from build123d import *

# Parameters (mm, degrees)
EXTRUDE_1_DEPTH     = 10
SKETCH_3_R          = 2
SKETCH_3_R_2        = 1.5
CUT_EXTRUDE_1_DEPTH = 30
CHAMFER_1_SIZE      = 5


with BuildPart() as part:
    # 草图1 → 凸台-拉伸1 (new body)
    with BuildSketch(Plane.XY):
        Polygon((0, 0), (35, 0), (35, -11), (62, -11), (62, -6), (45, -6), (45, 5), (0, 5), align=None)
    extrude(amount=EXTRUDE_1_DEPTH)

    # 草图3 → 切除-拉伸1 (cut)
    with BuildSketch(Plane.XZ.offset(11)):
        with Locations(Location((10, 5, 0), (0, 0, 270))):
            Circle(SKETCH_3_R)
        with Locations((57, 5)):
            Circle(SKETCH_3_R_2)
    extrude(amount=-CUT_EXTRUDE_1_DEPTH, mode=Mode.SUBTRACT)

    # 倒角1
    chamfer_1_edges = [part.edges().sort_by_distance(p)[0] for p in [
        (45, -6, 5),
        (35, 0, 5),
    ]]
    chamfer(chamfer_1_edges, length=CHAMFER_1_SIZE)


solid = part.part
Could you check a few things on this model? Use its own coordinates, in mm. A direction names the side the tool comes from. Coordinates: 2 decimals unless noted, no trailing zeros. Order: outer loops, then holes, each group sorted by start corner. A loop starts at its lowest first (then second) coordinate and runs counter-clockwise, first axis right, second up.
Q1. Suppose I cut it at B-B on z = 5. Please give me the cut outline in (x, y).
Q2. Suppose I cut it at A-A on x = 57. Please give me the cut outline in (y, z), and give its area (3 significant figures).
Q3. Will these pins go through, and if not, where does the flat tip stop? pin 1 (1.8 mm diameter, centred on y = -8.5, z = 7, fed in from -X); pin 2 (3 mm diameter, centred on x = 57, z = 6.5, fed in from +Y); pin 3 (1.5 mm diameter, centred on x = 13, z = 8, fed in from -Y).
Q4. Suppose I cut it at C-C on y = 3. Please give me the cut outline in (x, z), and give its area (3 significant figures).
Q5. Please list where these lines run through material, in increasing order: L1, parallel to Z at x = 57, y = -9.55; L2, parallel to Y at x = 15, z = 4.5; L3, parallel to Y at x = 57, z = 8.75.
Q6. Which directions (+Z, -Z, +X, -X, +Y, -Y) give clear straight access to the entire face, cutting with the end or side of a thin tool? Please do faces 5 (the flat face through (45, 2, 5)), 6 (the flat face through (48, -11, 5)), 7 (the flat face through (35, -8, 5)).
Q7. Thinking about a two-plate mould opening in X: for faces 1 (the cylindrical face through (58.43, -8.54, 5.45)), 2 (the flat face through (0, 3, 5)), 3 (the cylindrical face through (12, 2, 5)), 4 (the flat face through (55, -6, 5)), which applies, released by +X, released by -X, zero draft, split by the parting line, or undercut?
Q8. Suppose I cut it at D-D on z = 1. Please give me the cut outline in (x, y).
Answer:
1. outline: (0, 0) - (8, 0) - (8, 5) - (0, 5) - close; (12, 0) - (30, 0) - (35, -5) - (35, -11) - (55.5, -11) - (55.5, -6) - (50, -6) - (45, -1) - (45, 5) - (12, 5) - close; (58.5, -11) - (62, -11) - (62, -6) - (58.5, -6) - close
2. outline: (-11, 0) - (-6, 0) - (-6, 3.5) - (-11, 3.5) - close; (-11, 6.5) - (-6, 6.5) - (-6, 10) - (-11, 10) - close
2. area: 35.0 mm2
3. pin 1: stops at x = 35
3. pin 2: stops at y = -6
3. pin 3: stops at y = 0
4. outline: (0, 0) - (45, 0) - (45, 10) - (0, 10) - close; hole circle Ø4 at (10, 5)
4. area: 437 mm2
5. L1: z = 0 to 3.5, 6.5 to 10
5. L2: y = 0 to 5
5. L3: y = -11 to -6
6. face 5: +Z, -Z, +X, +Y
6. face 6: +Z, -Z, +X, -X, -Y
6. face 7: +Z, -Z, -X, -Y
7. face 1: undercut
7. face 2: released by -X
7. face 3: undercut
7. face 4: zero draft
8. outline: (0, 0) - (30, 0) - (35, -5) - (35, -11) - (62, -11) - (62, -6) - (50, -6) - (45, -1) - (45, 5) - (0, 5) - close
